from build123d import *

# Parameters (mm, degrees)
ESQUISSE1_W             = 80
ESQUISSE1_H             = 50
BOSS_EXTRU_1_DEPTH      = 40
CHANFREIN1_SIZE         = 30
CHANFREIN1_SIZE2        = 3.683536827
ESQUISSE2_R             = 12.5
ENL_V_MAT_EXTRU_1_DEPTH = 40


with BuildPart() as part:
    # Esquisse1 → Boss.-Extru.1 (new body)
    with BuildSketch(Plane(origin=(0, 0, 0), x_dir=(1, 0, 0), z_dir=(0, 1, 0))):
        Rectangle(ESQUISSE1_W, ESQUISSE1_H)
    extrude(amount=BOSS_EXTRU_1_DEPTH)

    # Chanfrein1
    chanfrein1_edges = [part.edges().sort_by_distance(p)[0] for p in [
        (-40, 40, 0),
    ]]
    chanfrein1_side = [part.faces().sort_by_distance(p)[0] for p in [
        (-40, 20, 0),
    ]]
    chamfer(chanfrein1_edges, length=CHANFREIN1_SIZE, length2=CHANFREIN1_SIZE2, reference=chanfrein1_side[0])

    # Esquisse2 → Enlèv. mat.-Extru.1 (cut)
    with BuildSketch(Plane(origin=(-40.615524004, 4.986959281, 0), x_dir=(0, 0, 1), z_dir=(-0.9925461516413225, 0.12186934340514435, 0))):
        with Locations(Location((0, 18.821046558, 0), (0, 0, 270))):
            Circle(ESQUISSE2_R)
    extrude(amount=-ENL_V_MAT_EXTRU_1_DEPTH, mode=Mode.SUBTRACT)


solid = part.part
Verification items for the finished model (mm, model axes). Round coordinates to 2 decimals unless told otherwise and drop trailing zeros. Write each loop counter-clockwise with the first axis right and the second up, starting at its lowest first coordinate (ties: lowest second). Pieces come first, ordered by that corner, then holes.
(1) Section check A-A (z = -20). Enter the section's corners in (x, y).
Returned:
outline: (-40, 0) - (40, 0) - (40, 40) - (-36.32, 40) - (-40, 10) - close
(2) Section check B-B (z = -5). Enter the section's corners in (x, y), plus the area to 3 significant figures.
Returned:
outline: (-40, 0) - (40, 0) - (40, 40) - (-36.32, 40) - (-36.93, 35.04) - (2.78, 30.16) - (-0.02, 7.42) - (-39.72, 12.3) - (-40, 10) - close
area: 2,230 mm2
(3) Mould release check, pull along Z, two halves, no side actions. Record for faces 1 (the flat face through (40, 20, 0)), 2 (the flat face through (1.4, 18.97, 0.18)), 3 (the cylindrical face through (-20.2, 9.43, 3.75)), 4 (the flat face through (-1, 20, -25)): pulls with the +Z half, pulls with the -Z half, needs draft (parallel to the pull), parting line crosses it, or undercut.
Returned:
face 1: needs draft
face 2: undercut
face 3: undercut
face 4: pulls with the -Z half
(4) Depth check by flat-ended pin: pin 1 Ø1 at (y, z) = (17.5, 16) entering from -X; pin 2 Ø1 at (x, z) = (22.5, -8.5) entering from -Y; pin 3 Ø1 at (y, z) = (24.5, 2) entering from -X. Enter the tip coordinate at first touch or a pass-through.
Returned:
pin 1: stops at x = -39.14
pin 2: stops at y = 0
pin 3: stops at x = 2.02
(5) Section check C-C (z = 11). Enter the section's corners in (x, y), plus the area to 3 significant figures.
Returned:
outline: (-40, 0) - (40, 0) - (40, 40) - (-36.32, 40) - (-37.6, 29.56) - (2.1, 24.69) - (0.66, 12.9) - (-39.05, 17.77) - (-40, 10) - close
area: 2,670 mm2
(6) Material ranges on line 1 (Z direction, x = -27, y = 29.5); line 2 (Z direction, x = -28.5, y = 16); line 3 (Y direction, x = -12, z = -1), recorded low to high.
Returned:
line 1: z = -25 to -10.24, 10.24 to 25
line 2: z = -25 to -10.73, 10.73 to 25
line 3: y = 0 to 7.88, 32.99 to 40
